Verification items for the finished model (mm, model axes). Give positions to 0.01 mm unless a question says otherwise; leave off trailing zeros. Loops run counter-clockwise (first coordinate to the right, second up) from the corner with the lowest first, then second, coordinate; pieces in that order, holes last. Notation, with made-up numbers: M -26.75,87 L 10.25,87 A35 cw 10.25,123 Z; hole C 35,57 d3. An arc over 180 degrees is marked long. Answer in a Markdown table with one row per item.
Autodesk Inventor part; units mm, degrees
ref_plane "Work Plane1" through (0, 0, 0) normal (0, 0, 1) x (1, 0, 0)
ref_plane "YZ Plane" through (0, 0, 0) normal (1, 0, 0) x (0, 1, 0)
ref_plane "XZ Plane" through (0, 0, 0) normal (0, 1, 0) x (-1, 0, 0)
ref_plane "Work Plane1" through (0, 0, 0) normal (0, 0, 1) x (1, 0, 0)
sketch "Sketch1" plane through (0, 0, 0) normal (0, 0, 1) x (1, 0, 0)
  circle A0 centre (0, 0) radius 14
  circle A1 centre (0, 0) radius 10
  line L0 (0, -14) -> (0, 14)
  point P0 (0, 10)
  point P1 (0, -10)
  dimension "d1" = 4
  dimension "d4" = 20
extrude "Extrusion1" add sketch "Sketch1" along normal mid plane 30 contours L0 A1 A0 picked at (-1.9145, -12.4342)
chamfer "Chamfer1" distance 3.175 angle 45 1 edges at (0, 14, 0)
properties part number "2101_Tx_Coil_Spacer_v1" material "Acetal Resin, White"
Item 1: Sectioned sample at A-A (z = -1.5). Record the cut outline in (x, y) (3 decimals).
Reported:
| item | result |
|---|---|
| outline | M -3.155,13.64 A14 ccw 0,-14 L 0,-10 A10 cw 0,10 L 0,10.825 Z |
Item 2: Sectioned sample at C-C (y = 5). Record the cut outline in (x, z), and give its area (3 significant figures).
Reported:
| item | result |
|---|---|
| outline | M -13.08,-15 L -8.66,-15 L -8.66,15 L -13.08,15 Z |
| area | 132 mm^2 |
Item 3: Scan lines: L1, parallel to Y at x = -1.5, z = 5.5; L2, parallel to Y at x = -5, z = 11; L3, parallel to X at y = 1.5, z = 13.5. Record each from-to range of solid material in increasing order. Write a range as [from, to].
Reported:
| item | result |
|---|---|
| L1 | y = [-13.92, -9.89], [9.89, 12.16] |
| L2 | y = [-13.08, -8.66], [8.66, 13.08] |
| L3 | x = [-13.92, -9.89] |
Item 4: Sectioned sample at B-B (y = 0). Record the cut outline in (x, z), and give its area (3 significant figures).
Reported:
| item | result |
|---|---|
| outline | M -14,-15 L -10,-15 L -10,15 L -14,15 Z |
| area | 120 mm^2 |
Item 5: Go/stop test with flat-tipped pins: pin 1 (1 mm diameter, centred on x = -5.5, z = -9, fed in from -Y); pin 2 (6 mm diameter, centred on x = -6.5, z = 10.5, fed in from -Y); pin 3 (4 mm diameter, centred on y = 1.5, z = -4.5, fed in from +X). Record where each tip stops, or that it passes through.
Reported:
| item | result |
|---|---|
| pin 1 | stops at y = -13.08 |
| pin 2 | stops at y = -13.56 |
| pin 3 | stops at x = -9.37 |
Item 6: Release check for a two-part mould opening along Y. For faces 1 (the flat face through (0, -12, 0)), 2 (the cylindrical face through (-13.874, -1.871, -0.21)), 3 (the cylindrical face through (-10, 0, 0)) record: released by +Y, released by -Y, zero draft, split by the parting line, or undercut.
Reported:
| item | result |
|---|---|
| face 1 | zero draft |
| face 2 | split by the parting line |
| face 3 | undercut |
